Input: part model. Units: mm. Frame: model coordinates. Face numbers are marked on the shaded views. A direction names the side the tool comes from. Coordinates: 2 decimals unless noted, no trailing zeros. Write each loop counter-clockwise with the first axis right and the second up, starting at its lowest first coordinate (ties: lowest second). Pieces come first, ordered by that corner, then holes. Notation, with made-up numbers: (18.25, -30.75) -> (71.25, -30.75) arc R31 ccw to (71.25, -5.75) -> close; hole circle Ø9 at (85.25, 84). An arc over 180 degrees is marked (long way). Use one line per item in the form item = value. Start each with the question number.
(1) Cut plane B-B on y = 69.5. State how many separate pieces and enclosed holes the cut face has, plus the area to 3 significant figures.
(2) Set-up query: the marked faces 4, 5 and 6. Return all of +Z, -Z, +X, -X, +Y, -Y with unobstructed straight access to the full face (end or side cutting, diameter ignored); none if empty.
(3) Ray query, line 1 along X through (y, z) = (107, 237.5); line 2 along Z through (x, y) = (63, 46) (3 decimals); line 3 along Y through (x, z) = (201, 156.5). Return the intervals inside material, ascending.
(4) Cut plane C-C on z = 208. Return the cut outline in (x, y).
(5) Cut plane D-D on x = 125. Return the cut outline in (y, z) (1 decimal).
(6) Pull-direction query (Z, two-part tool) for the marked faces 1, 2 and 3; classes: released by +Z, released by -Z, zero draft, split by the parting line, or undercut.
(7) First-contact query: pin 1 (5 mm diameter, centred on y = 96, z = 202.5, fed in from -X); pin 2 (4.5 mm diameter, centred on y = 72, z = 349, fed in from -X); pin 3 (12 mm diameter, centred on y = 71, z = 348, fed in from +X). Flat tips, straight axial feed; report the tip coordinate or a pass-through.
```python
from build123d import *

# Parameters (mm, degrees)
SKETCH1_W           = 222.25
SKETCH1_H           = 63.5
BOSS_EXTRUDE1_DEPTH = 377.825
SKETCH2_W           = 25.4
SKETCH2_H           = 428.625
BOSS_EXTRUDE2_DEPTH = 50.8
SKETCH3_W           = 132.08
SKETCH3_H           = 149.86
BOSS_EXTRUDE3_DEPTH = 50.8
SKETCH4_W           = 101.6
SKETCH4_H           = 76.2
BOSS_EXTRUDE4_DEPTH = 25.4
SKETCH5_W           = 78.778649954
SKETCH5_H           = 46.015700821
BOSS_EXTRUDE5_DEPTH = 15.24
CUT_EXTRUDE1_DEPTH  = 127


with BuildPart() as part:
    # Sketch1 → Boss-Extrude1 (new body)
    with BuildSketch(Plane.XY):
        with Locations((111.125, 31.75)):
            Rectangle(SKETCH1_W, SKETCH1_H)
    extrude(amount=BOSS_EXTRUDE1_DEPTH)

    # Sketch2 → Boss-Extrude2 (add)
    with BuildSketch(Plane(origin=(0, 63.5, 0), x_dir=(1, 0, 0), z_dir=(0, 1, 0))):
        with Locations((158.75, -188.9125)):
            Rectangle(SKETCH2_W, SKETCH2_H)
    extrude(amount=BOSS_EXTRUDE2_DEPTH)

    # Sketch3 → Boss-Extrude3 (add)
    with BuildSketch(Plane(origin=(0, 63.5, 0), x_dir=(1, 0, 0), z_dir=(0, 1, 0))):
        with Locations((72.39, -188.9125)):
            Rectangle(SKETCH3_W, SKETCH3_H)
    extrude(amount=BOSS_EXTRUDE3_DEPTH)

    # Sketch4 → Boss-Extrude4 (add)
    with BuildSketch(Plane(origin=(0, 63.5, 0), x_dir=(1, 0, 0), z_dir=(0, 1, 0))):
        with Locations((69.606671705, -56.197197529)):
            Rectangle(SKETCH4_W, SKETCH4_H)
    extrude(amount=BOSS_EXTRUDE4_DEPTH)

    # Sketch5 → Boss-Extrude5 (add)
    with BuildSketch(Plane(origin=(0, 63.5, 0), x_dir=(1, 0, 0), z_dir=(0, 1, 0))):
        with Locations((69.91393095, -338.241458835)):
            Rectangle(SKETCH5_W, SKETCH5_H)
    extrude(amount=BOSS_EXTRUDE5_DEPTH)

    # Sketch8 → Cut-Extrude1 (cut)
    with BuildSketch(Plane(origin=(0, 114.3, 0), x_dir=(1, 0, 0), z_dir=(0, 1, 0))):
        Polygon((171.45, 25.4), (146.05, 0), (146.05, 25.4), align=None)
        Polygon((171.45, -403.225), (146.05, -377.825), (146.05, -403.225), align=None)
    extrude(amount=-CUT_EXTRUDE1_DEPTH, mode=Mode.SUBTRACT)


solid = part.part
```
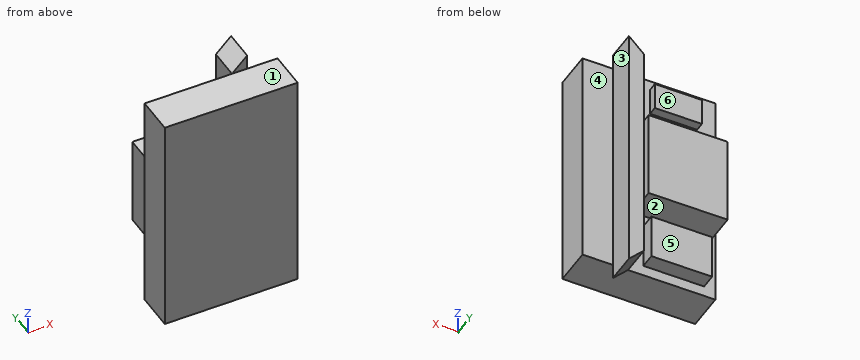
Values:
q1.separate_pieces = 4
q1.enclosed_holes = 0
q1.area = 41,400 mm2
q2.face_4 = +Z, -Z, +X, +Y
q2.face_5 = -Z, -X, +Y
q2.face_6 = +Z, -X, +Y
q3.line_1 = 6.35 to 138.43, 146.05 to 171.45
q3.line_2 = 0 to 377.825
q3.line_3 = 0 to 63.5
q4.outline = (0, 0) -> (222.25, 0) -> (222.25, 63.5) -> (171.45, 63.5) -> (171.45, 114.3) -> (146.05, 114.3) -> (146.05, 63.5) -> (138.43, 63.5) -> (138.43, 114.3) -> (6.35, 114.3) -> (6.35, 63.5) -> (0, 63.5) -> close
q5.outline = (0, 0) -> (63.5, 0) -> (63.5, 114) -> (114.3, 114) -> (114.3, 263.8) -> (63.5, 263.8) -> (63.5, 377.8) -> (0, 377.8) -> close
q6.face_1 = released by +Z
q6.face_2 = undercut
q6.face_3 = zero draft
q7.pin_1 = 6.35
q7.pin_2 = 30.52
q7.pin_3 = 171.45
